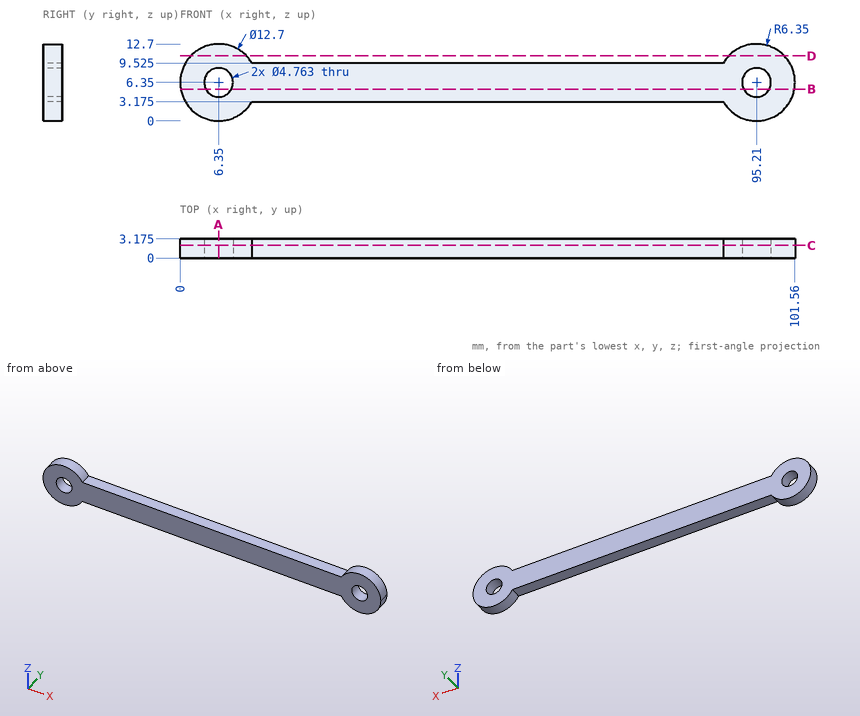
Could you check a few things on this drawing? It's one solid part, dimensions in mm from its lowest x, y, z. Coordinates: 2 decimals unless noted, no trailing zeros. Loops run counter-clockwise (first coordinate to the right, second up) from the corner with the lowest first, then second, coordinate; pieces in that order, holes last.
1. Imagine slicing it at D-D (z = 10.75). Please give me the cut outline in (x, y) (1 decimal).
2. Imagine slicing it at A-A (x = 6.35). Please give me the cut outline in (y, z) (1 decimal).
3. I need wall thicknesses on L1, parallel to X at y = 2.65, z = 6.5; L2, parallel to X at y = 0.65, z = 7.75 (1 decimal); L3, parallel to Z at x = 38, y = 1.8 (1 decimal). Which ranges of each line are inside material? Lowest first, please.
4. Imagine slicing it at C-C (y = 2.1). Give the number of separate pieces and of enclosed holes in the cut face, and give its area (3 significant figures).
5. For P1, Ø1, axis at x = 51.5, y = 2, coming from the +Z side (1 decimal); P2, Ø1.6, axis at x = 61, y = 2, coming from the -Z side (1 decimal); P3, Ø1, axis at y = 2, z = 10.5, coming from the -X side (1 decimal), each with a flat end and sliding along its axis, tell me the tip position at first contact or that it passes through.
6. Imagine slicing it at B-B (z = 5.25). Please give me the cut outline in (x, y) (1 decimal).
Computed values:
1. outline: (1.8, 0) - (10.9, 0) - (10.9, 3.2) - (1.8, 3.2) - close; (90.6, 0) - (99.8, 0) - (99.8, 3.2) - (90.6, 3.2) - close
2. outline: (0, 0) - (3.2, 0) - (3.2, 4) - (0, 4) - close; (0, 8.7) - (3.2, 8.7) - (3.2, 12.7) - (0, 12.7) - close
3. L1: x = 0 to 3.97, 8.73 to 92.83, 97.59 to 101.56
3. L2: x = 0.2 to 4.4, 8.3 to 93.3, 97.1 to 101.4
3. L3: z = 3.2 to 9.5
4. separate pieces: 1
4. enclosed holes: 2
4. area: 705 mm2
5. P1: stops at z = 9.5
5. P2: stops at z = 3.2
5. P3: stops at x = 1.2
6. outline: (0.1, 0) - (4.2, 0) - (4.2, 3.2) - (0.1, 3.2) - close; (8.5, 0) - (93.1, 0) - (93.1, 3.2) - (8.5, 3.2) - close; (97.3, 0) - (101.5, 0) - (101.5, 3.2) - (97.3, 3.2) - close
